Verification items for this drawing (mm, ordinates from the low corner). Round coordinates to 2 decimals unless told otherwise and drop trailing zeros. Order: outer loops, then holes, each group sorted by start corner. A loop starts at its lowest first (then second) coordinate and runs counter-clockwise, first axis right, second up. Notation, with made-up numbers: M 68.5,-2.75 L 78.5,-2.75 A19 cw 78.5,10.25 Z; hole C 9,72.25 d3. An arc over 180 degrees is marked long. Return JSON: item names as keys, results as strings. Group by question number.
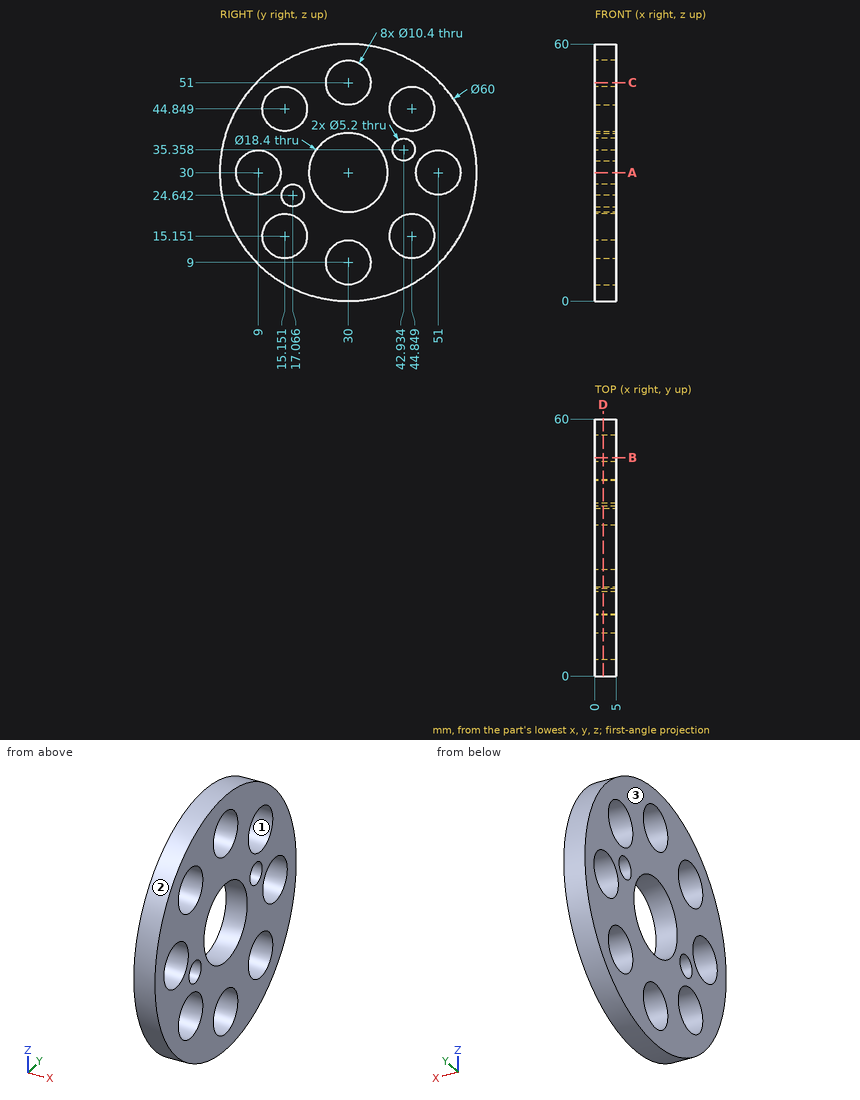
1. Thickness scan on line 1 along Y through (x, z) = (2.05, 23); line 2 along Z through (x, y) = (4.7, 16) (1 decimal); line 3 along Y through (x, z) = (0.5, 32.5) (1 decimal). Record the ranges inside material, lowest first. Write a range as from..to.
2. Cross-section at D-D (x = 1.95). Give the number of separate pieces and of enclosed holes in the cut face, plus the area to 3 significant figures.
3. Go/stop test with flat-tipped pins: pin 1 (3 mm diameter, centred on x = 0.5, y = 36, fed in from +Z); pin 2 (1.5 mm diameter, centred on x = 3, z = 48.5, fed in from -Y) (1 decimal); pin 3 (6 mm diameter, centred on y = 30, z = 9, fed in from +X); pin 4 (1 mm diameter, centred on x = 3, z = 17, fed in from +Y). Record where each tip stops, or that it passes through.
4. Draft check along Z on the marked faces 1, 2 and 3. Enter one of: +Z half, -Z half, draft (parallel to the pull), parting line (faces both ways), or undercut.
5. Cross-section at B-B (y = 51). Enter the section's corners in (x, z) (1 decimal).
6. Cross-section at A-A (z = 30). Enter the section's corners in (x, y), plus the area to 3 significant figures.
Computed:
{
 "1": {"line 1": "y = 0.83..15.05, 19.08..24.03, 35.97..59.17", "line 2": "z = 3.5..10, 20.3..22.3, 27..39.7, 50..56.5", "line 3": "y = 0.1..4.4, 13.6..21.1, 38.9..46.4, 55.6..59.9"},
 "2": {"separate pieces": "1", "enclosed holes": "11", "area": "1,840 mm²"},
 "3": {"pin 1": "stops at z = 59.66", "pin 2": "stops at y = 5.8", "pin 3": "passes through", "pin 4": "stops at y = 57.27"},
 "4": {"face 1": "undercut", "face 2": "parting line", "face 3": "draft"},
 "5": {"outline": "M 0,8.6 L 5,8.6 L 5,24.8 L 0,24.8 Z; M 0,35.2 L 5,35.2 L 5,51.4 L 0,51.4 Z"},
 "6": {"outline": "M 0,0 L 5,0 L 5,3.8 L 0,3.8 Z; M 0,14.2 L 5,14.2 L 5,20.8 L 0,20.8 Z; M 0,39.2 L 5,39.2 L 5,45.8 L 0,45.8 Z; M 0,56.2 L 5,56.2 L 5,60 L 0,60 Z", "area": "104 mm²"}
}
